```python
from build123d import *

# Parameters (mm, degrees)
SKETCH2_W           = 320
SKETCH2_H           = 320
BOSS_EXTRUDE1_DEPTH = 10


with BuildPart() as part:
    # Sketch2 → Boss-Extrude1 (new, symmetric)
    with BuildSketch(Plane.XY):
        Polygon((160, -230), (160, -180), (-160, -180), (-160, -230), (-180, -230), (-180, 180), (180, 180), (180, -230), align=None)
        Rectangle(SKETCH2_W, SKETCH2_H, mode=Mode.SUBTRACT)
    extrude(amount=BOSS_EXTRUDE1_DEPTH, both=True)


solid = part.part
```
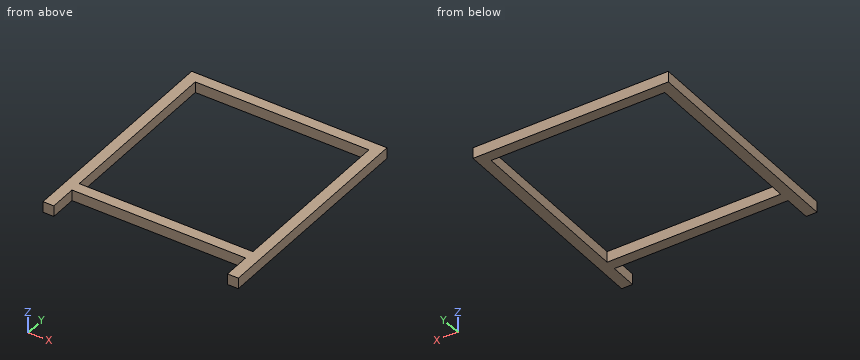
Input: part model. Units: mm. Frame: model coordinates. Give positions to 0.01 mm unless a question says otherwise; leave off trailing zeros. Loops run counter-clockwise (first coordinate to the right, second up) from the corner with the lowest first, then second, coordinate; pieces in that order, holes last. Notation, with made-up numbers: (-25.5, 82.5) -> (23.5, 82.5) arc R26 ccw to (23.5, 116.5) -> close; hole circle Ø6 at (67.25, 14). An arc over 180 degrees is marked (long way). Use a Markdown table: item, result.
Q1. Section query C-C, the plane z = -6.25. Return the cut outline in (x, y), plus the area to 3 significant figures.
Entries:
| item | result |
|---|---|
| outline | (-180, -230) -> (-160, -230) -> (-160, -180) -> (160, -180) -> (160, -230) -> (180, -230) -> (180, 180) -> (-180, 180) -> close; hole (-160, -160) -> (160, -160) -> (160, 160) -> (-160, 160) -> close |
| area | 29,200 mm² |
Q2. Section query A-A, the plane x = -127.5. Return the cut outline in (y, z), plus the area to 3 significant figures.
Entries:
| item | result |
|---|---|
| outline | (-180, -10) -> (-160, -10) -> (-160, 10) -> (-180, 10) -> close; (160, -10) -> (180, -10) -> (180, 10) -> (160, 10) -> close |
| area | 800 mm² |
Q3. Ray query, probe 1 along X at (y, z) = (158.5, 5.25). Return the intervals inside material, ascending. Write a range as from..to.
Entries:
| item | result |
|---|---|
| probe 1 | x = -180..-160, 160..180 |
Q4. First-contact query: P1, Ø10, axis at x = 63, z = 6, coming from the -Y side. Flat tip, straight axial feed; report the tip coordinate or a pass-through.
Entries:
| item | result |
|---|---|
| P1 | stops at y = -180 |
